Here's how the part is built. I have some questions about the finished solid (model axes, mm). A direction names the side the tool comes from. Give positions to 0.01 mm unless a question says otherwise; leave off trailing zeros. Loops run counter-clockwise (first coordinate to the right, second up) from the corner with the lowest first, then second, coordinate; pieces in that order, holes last.
Q1. I need wall thicknesses on probe 1 along X at (y, z) = (-5.5, 10) (3 decimals); probe 2 along Z at (x, y) = (62, -12.7); probe 3 along Z at (x, y) = (50, 3.5). Which ranges of each line are inside material? Lowest first, please.
Q2. I'm going to push flat-ended pins straight in: P1, Ø15.5, axis at x = -54, y = 5, coming from the +Z side; P2, Ø8, axis at x = -9.5, z = 39.5, coming from the -Y side; P3, Ø1, axis at y = 20, z = 28.5, coming from the -X side. Where does each tip first touch, or does it pass through?
Q3. For faces 1 (the face through (0, 25.4, 44)), 2 (the face through (6, 10, 45.085)), 3 (the face through (54, 11, 25.4)), 4 (the face through (-54, 10, 25.4)), 5 (the face through (0, 0, 43)), which set-ups out of +Z, -Z, +X, -X, +Y, -Y let a thin tool reach every point of the face, with its end or its side?
Q4. Suppose I cut it at C-C (y = 4.5). List the corners of the cut face in (x, z) for me (3 decimals).
Q5. Suppose I cut it at A-A (y = 17). List the corners of the cut face in (x, z) for me (3 decimals), and give its area (3 significant figures).
Q6. Thinking about a two-plate mould opening in Z: for faces 6 (the face through (-57.785, -6.9, 9.7)), 7 (the face through (-60.916, -9.286, 18.054)), 8 (the face through (36.25, 12.52, 36.49)), 9 (the face through (-6, 10, 41.426)), which applies, pulls with the +Z half, pulls with the -Z half, needs draft (parallel to the pull), parting line crosses it, or undercut?
Q7. Suppose I cut it at D-D (x = 14.5). List the corners of the cut face in (y, z) for me (3 decimals), and give its area (3 significant figures).
Q8. Suppose I cut it at B-B (z = 35). List the corners of the cut face in (x, y) for me, and give its area (3 significant figures).
```python
from build123d import *

# Parameters (mm, degrees)
F0_W     = 6.35
F0_H     = 25.4
F1_DEPTH = 25.4
F2_DEPTH = 25.4
F3_R     = 6.35
F4_DEPTH = 76.2
F7_DEPTH = 76.2


with BuildPart() as f1:
    # F0 (on Front) → F1 (new body)
    with BuildSketch(Plane.XZ):
        with BuildLine():
            Line((-44.7294, 18.1192818743), (-44.7294, 25.3937000187))
            ThreePointArc((-44.7294, 25.3937000187), (-49.7303524721, 13.13207021), (-51.435, 0))
            Line((-51.435, 0), (-48.26, 0))
            ThreePointArc((-48.26, 0), (-47.3691273088, 9.2300258938), (-44.7294, 18.1192818743))
        make_face()
        with BuildLine():
            ThreePointArc((-51.435, 0), (-49.7303524721, 13.13207021), (-44.7294, 25.3937000187))
            Line((-44.7294, 25.3937000187), (-44.7294, 25.4))
            Line((-44.7294, 25.4), (-51.435, 25.4))
            Line((-51.435, 25.4), (-51.435, 0))
        make_face()
        with Locations((-54.61, 12.7)):
            Rectangle(F0_W, F0_H)
        with Locations((-60.96, 12.7)):
            Rectangle(F0_W, F0_H)
        with BuildLine():
            ThreePointArc((44.7294, 25.3937000187), (36.1112423463, 36.6270037159), (24.7568576358, 45.085))
            Line((24.7568576358, 45.085), (24.7568576358, 41.426146333))
            ThreePointArc((24.7568576358, 41.426146333), (36.6454292209, 31.4028679776), (44.7294, 18.1192818743))
            Line((44.7294, 18.1192818743), (44.7294, 25.3937000187))
        make_face()
        with BuildLine():
            ThreePointArc((51.435, 0), (49.7303524721, 13.13207021), (44.7294, 25.3937000187))
            Line((44.7294, 25.3937000187), (44.7294, 18.1192818743))
            ThreePointArc((44.7294, 18.1192818743), (47.3691273088, 9.2300258938), (48.26, 0))
            Line((48.26, 0), (51.435, 0))
        make_face()
        with BuildLine():
            Line((44.7294, 25.4), (44.7294, 25.3937000187))
            ThreePointArc((44.7294, 25.3937000187), (49.7303524721, 13.13207021), (51.435, 0))
            Line((51.435, 0), (51.435, 25.4))
            Line((51.435, 25.4), (44.7294, 25.4))
        make_face()
        with Locations((54.61, 12.7)):
            Rectangle(F0_W, F0_H)
        with Locations((60.96, 12.7)):
            Rectangle(F0_W, F0_H)
        with BuildLine():
            Line((-24.7568576358, 41.426146333), (-24.7568576358, 45.085))
            ThreePointArc((-24.7568576358, 45.085), (-36.1112423463, 36.6270037159), (-44.7294, 25.3937000187))
            Line((-44.7294, 25.3937000187), (-44.7294, 18.1192818743))
            ThreePointArc((-44.7294, 18.1192818743), (-36.6454292209, 31.4028679776), (-24.7568576358, 41.426146333))
        make_face()
        with BuildLine():
            ThreePointArc((24.7568576358, 41.426146333), (21.0657218153, 43.419614973), (17.2154109739, 45.085))
            Line((17.2154109739, 45.085), (0, 45.085))
            Line((0, 45.085), (-17.2154109739, 45.085))
            ThreePointArc((-17.2154109739, 45.085), (-21.0657218153, 43.419614973), (-24.7568576358, 41.426146333))
            Line((-24.7568576358, 41.426146333), (24.7568576358, 41.426146333))
        make_face()
        with BuildLine():
            Line((-17.2154109739, 45.085), (-24.7568576358, 45.085))
            Line((-24.7568576358, 45.085), (-24.7568576358, 41.426146333))
            ThreePointArc((-24.7568576358, 41.426146333), (-21.0657218153, 43.419614973), (-17.2154109739, 45.085))
        make_face()
        with BuildLine():
            Line((24.7568576358, 41.426146333), (24.7568576358, 45.085))
            Line((24.7568576358, 45.085), (17.2154109739, 45.085))
            ThreePointArc((17.2154109739, 45.085), (21.0657218153, 43.419614973), (24.7568576358, 41.426146333))
        make_face()
    extrude(amount=-F1_DEPTH)

    # F0 (on Front) → F2 (join)
    with BuildSketch(Plane.XZ):
        with Locations((60.96, 12.7)):
            Rectangle(F0_W, F0_H)
        with Locations((-60.96, 12.7)):
            Rectangle(F0_W, F0_H)
    extrude(amount=F2_DEPTH)


with BuildPart() as f4:
    # F3 (on Right) → F4 (new body, symmetric)
    with BuildSketch(Plane.YZ):
        with Locations((-12.7, 12.7)):
            Circle(F3_R)
    extrude(amount=F4_DEPTH, both=True)


with BuildPart() as f4b:
    # F3 (on Right) → F4, piece 2 (new body, symmetric)
    with BuildSketch(Plane.YZ):
        with BuildLine():
            ThreePointArc((-25.4, 12.7), (-21.6802561211, 21.6802561211), (-12.7, 25.4))
            Line((-12.7, 25.4), (-25.4, 25.4))
            Line((-25.4, 25.4), (-25.4, 12.7))
        make_face()
    extrude(amount=F4_DEPTH, both=True)


with BuildPart() as f4c:
    # F3 (on Right) → F4, piece 3 (new body, symmetric)
    with BuildSketch(Plane.YZ):
        with BuildLine():
            Line((-25.4, 0), (-12.7, 0))
            ThreePointArc((-12.7, 0), (-21.6802561211, 3.7197438789), (-25.4, 12.7))
            Line((-25.4, 12.7), (-25.4, 0))
        make_face()
    extrude(amount=F4_DEPTH, both=True)


with BuildPart() as f1_1:
    add(f1.part)

    # F5: cut F4b, F4, F4c
    add(f4b.part, mode=Mode.SUBTRACT)
    add(f4.part, mode=Mode.SUBTRACT)
    add(f4c.part, mode=Mode.SUBTRACT)


with BuildPart() as f7:
    # F6 (on Top) → F7 (new body)
    with BuildSketch(Plane.XY):
        with BuildLine():
            ThreePointArc((0, 6.35), (4.4901280605, 8.2098719395), (6.35, 12.7))
            ThreePointArc((6.35, 12.7), (-4.4901280605, 17.1901280605), (0, 6.35))
        make_face()
    extrude(amount=F7_DEPTH)


with BuildPart() as f1_2:
    add(f1_1.part)

    # F8: cut F7
    add(f7.part, mode=Mode.SUBTRACT)


solid = f1_2.part
```
Solutions:
1. probe 1: x = -64.135 to -57.785, 57.785 to 64.135
1. probe 2: z = 0 to 6.35, 19.05 to 25.4
1. probe 3: z = 0 to 25.4
2. P1: stops at z = 25.4
2. P2: stops at y = 0
2. P3: stops at x = -43.15
3. face 1: +Z, -Z, +X, -X, +Y
3. face 2: +Z, +X, -X, +Y, -Y
3. face 3: +Z, +X, +Y, -Y
3. face 4: +Z, -X, +Y, -Y
3. face 5: +Z, -Z, -Y
4. outline: (-64.135, 0) - (-48.26, 0) arc R48.26 cw to (-24.757, 41.426) - (24.757, 41.426) arc R48.26 cw to (48.26, 0) - (64.135, 0) - (64.135, 25.4) - (44.729, 25.4) - (44.729, 25.394) arc R51.435 ccw to (24.757, 45.085) - (-24.757, 45.085) arc R51.435 ccw to (-44.729, 25.394) - (-44.729, 25.4) - (-64.135, 25.4) - close
5. outline: (-64.135, 0) - (-48.26, 0) arc R48.26 cw to (-24.757, 41.426) - (-4.673, 41.426) - (-4.673, 45.085) - (-24.757, 45.085) arc R51.435 ccw to (-44.729, 25.394) - (-44.729, 25.4) - (-64.135, 25.4) - close; (4.673, 41.426) - (24.757, 41.426) arc R48.26 cw to (48.26, 0) - (64.135, 0) - (64.135, 25.4) - (44.729, 25.4) - (44.729, 25.394) arc R51.435 ccw to (24.757, 45.085) - (4.673, 45.085) - close
5. area: 1,240 mm2
6. face 6: needs draft
6. face 7: undercut
6. face 8: pulls with the +Z half
6. face 9: pulls with the -Z half
7. outline: (0, 41.426) - (25.4, 41.426) - (25.4, 45.085) - (0, 45.085) - close
7. area: 92.9 mm2
8. outline: (-37.69, 0) - (-33.23, 0) - (-33.23, 25.4) - (-37.69, 25.4) - close; (33.23, 0) - (37.69, 0) - (37.69, 25.4) - (33.23, 25.4) - close
8. area: 227 mm2
